Could you check a few things on this model? Use its own coordinates, in mm. Give positions to 0.01 mm unless a question says otherwise; leave off trailing zeros. Write each loop counter-clockwise with the first axis right and the second up, starting at its lowest first coordinate (ties: lowest second). Pieces come first, ordered by that corner, then holes. Notation, with made-up numbers: (-38.75, 37) -> (-10.75, 37) arc R16 ccw to (-10.75, 61) -> close; hole circle Ø2 at (-14, -37.75). An arc over 180 degrees is marked (long way). One line per question, with ' | ' between items.
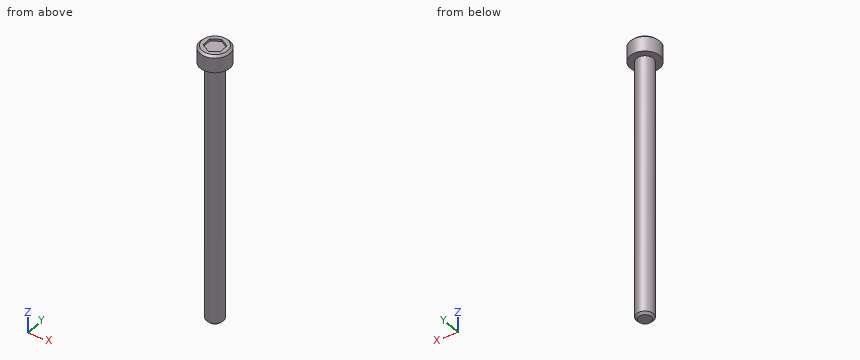
Autodesk Inventor part; units mm, degrees
ref_plane "YZ Plane" through (0, 0, 0) normal (1, 0, 0) x (0, 1, 0)
ref_plane "XZ Plane" through (0, 0, 0) normal (0, 1, 0) x (-1, 0, 0)
ref_plane "XY Plane" through (0, 0, 0) normal (0, 0, 1) x (1, 0, 0)
sketch "Sketch1" plane through (0, 0, 0) normal (0, 0, 1) x (1, 0, 0)
  circle A0 centre (0, 0) radius 3.5
  dimension "d0" = 7
extrude "Extrusion1" add sketch "Sketch1" along normal blind 4
sketch "Sketch2" plane through (0, 0, 0) normal (0, 0, 1) x (1, 0, 0)
  circle A0 centre (0, 0) radius 2
  dimension "d3" = 4
extrude "Extrusion2" add sketch "Sketch2" against normal blind 62
chamfer "Chamfer1" distance 0.5 angle 45 2 edges at (-3.5, 0, 4) (-2, 0, -62)
sketch "Sketch3" plane through (0, 0, 4) normal (0, 0, 1) x (1, 0, 0)
  circle A0 centre (0, 0) radius 2
  line L0 (-2, 1.1547) -> (0, 2.3094)
  line L1 (0, 2.3094) -> (2, 1.1547)
  line L2 (2, 1.1547) -> (2, -1.1547)
  line L3 (2, -1.1547) -> (0, -2.3094)
  line L4 (0, -2.3094) -> (-2, -1.1547)
  line L5 (-2, -1.1547) -> (-2, 1.1547)
  point P0 (-2, 0)
extrude "Extrusion3" cut sketch "Sketch3" against normal blind 0.5
properties part number "bolt"
Q1. Imagine slicing it at A-A on y = 0. Please give me the cut outline in (x, z).
Answer below:
outline: (-3.5, 0) -> (-2, 0) -> (-2, -61.5) -> (-1.5, -62) -> (1.5, -62) -> (2, -61.5) -> (2, 0) -> (3.5, 0) -> (3.5, 3.5) -> (3, 4) -> (2, 4) -> (2, 3.5) -> (-2, 3.5) -> (-2, 4) -> (-3, 4) -> (-3.5, 3.5) -> close
Q2. Imagine slicing it at B-B on z = -8. Please give me the cut outline in (x, y).
Answer below:
outline: circle Ø4 at (0, 0)
Q3. Will these pins go through, and if not, where does the flat tip stop? pin 1 (3 mm diameter, centred on x = -0.5, z = -42.5, fed in from +Y); pin 2 (1 mm diameter, centred on x = 1, y = -1, fed in from +Z).
Answer below:
pin 1: stops at y = 2 | pin 2: stops at z = 3.5
Q4. If I drill on line 1 along Z through (x, y) = (-2.25, 1.25); line 2 along X through (y, z) = (-0.75, -23); line 3 along Z through (x, y) = (0.75, -3), over which ranges is the centre line in solid material (lowest first)?
Answer below:
line 1: z = 0 to 4 | line 2: x = -1.85 to 1.85 | line 3: z = 0 to 3.91
